The listing builds one solid part. Answer for the finished solid, in the listing's coordinates (mm). Face numbers are marked on the shaded views. Give positions to 0.01 mm unless a question says otherwise; leave off trailing zeros. Loops run counter-clockwise (first coordinate to the right, second up) from the corner with the lowest first, then second, coordinate; pieces in that order, holes last. Notation, with made-up numbers: M -6.75,24 L 7.25,24 A31 cw 7.25,58 Z; hole C 3.5,40 d2. An arc over 180 degrees is marked long. One line per item, written item: value. Start each with the question number.
Q1. A cutting plane is placed at B-B, the plane z = -408. Determine the outline of the cut face in (x, y).
Q2. The mould has two halves that part along Y. Classify the marked faces 1 and 2: +Y half, -Y half, draft (parallel to the pull), parting line (faces both ways), or undercut.
Q3. Flat-ended cylindrical pins translate along their axes: pin 1 (9 mm diameter, centred on y = -4.5, z = -219, fed in from -X); pin 2 (8 mm diameter, centred on y = 5, z = 227, fed in from +X); pin 3 (8 mm diameter, centred on x = -15, y = -13.5, fed in from +Z). Find the tip coordinate at first contact, or state that the pin passes through.
Q4. A cutting plane is placed at C-C, the plane y = 8.5. Determine the outline of the cut face in (x, z).
Q5. Consider L1, parallel to Y at x = -43.5, z = 124.5; L2, parallel to X at y = -5, z = 169. Determine where each line is inside the solid, lowest interval first.
Q6. A cutting plane is placed at A-A, the plane x = -23.5. Determine the outline of the cut face in (y, z).
from build123d import *

# Parameters (mm, degrees)
SALIENTE_EXTRUIR1_DEPTH = 500


with BuildPart() as part:
    # Croquis1 → Saliente-Extruir1 (new, symmetric)
    with BuildSketch(Plane.XY):
        Polygon((50, 19.7625), (0, 19.7625), (0, 0), (4.7625, 0), (4.7625, 15), (50, 15), align=None)
        Polygon((4.7625, 0), (0, 0), (0, -19.7625), (50, -19.7625), (50, -15), (4.7625, -15), align=None)
        Polygon((0, 0), (0, 19.7625), (-50, 19.7625), (-50, 15), (-4.7625, 15), (-4.7625, 0), align=None)
        Polygon((0, -19.7625), (0, 0), (-4.7625, 0), (-4.7625, -15), (-50, -15), (-50, -19.7625), align=None)
    extrude(amount=SALIENTE_EXTRUIR1_DEPTH, both=True)


solid = part.part
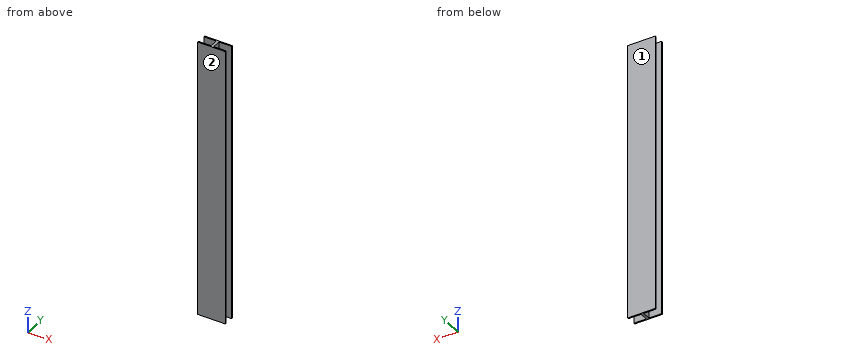
Answer block:
1. outline: M -50,-19.76 L 50,-19.76 L 50,-15 L 4.76,-15 L 4.76,15 L 50,15 L 50,19.76 L -50,19.76 L -50,15 L -4.76,15 L -4.76,-15 L -50,-15 Z
2. face 1: +Y half
2. face 2: -Y half
3. pin 1: x = -4.76
3. pin 2: x = 4.76
3. pin 3: z = 500
4. outline: M -4.76,-500 L 4.76,-500 L 4.76,500 L -4.76,500 Z
5. L1: -19.76 to -15, 15 to 19.76
5. L2: -4.76 to 4.76
6. outline: M -19.76,-500 L -15,-500 L -15,500 L -19.76,500 Z; M 15,-500 L 19.76,-500 L 19.76,500 L 15,500 Z
